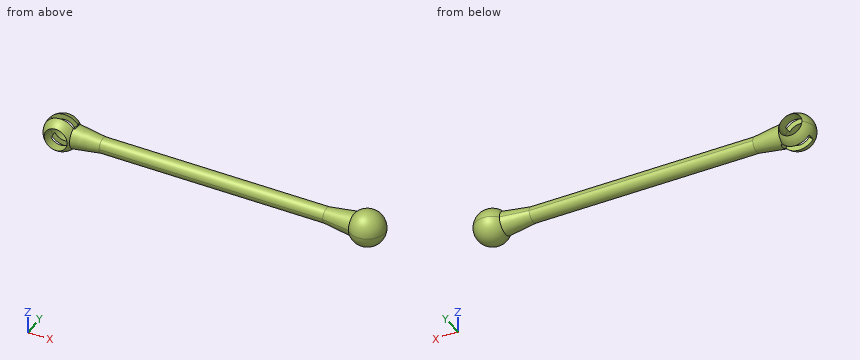
```python
from build123d import *
from build123d import SkipClean  # not in build123d's __all__

# Parameters (mm, degrees)
F2_W           = 30
F2_H           = 1.5
F3_ANGLE_BACK  = 90
F3_ANGLE       = 180
F5_ANGLE_BACK  = 90
F5_ANGLE       = 180
F7_ANGLE_BACK  = 90
F7_ANGLE       = 180
F9_R           = 2.25
F10_DEPTH      = 3.401
F10_DEPTH_BACK = 3.401
F12_DEPTH      = 0.75


with BuildPart() as f3:
    # F2 (on Front) → F3 (revolve)
    with BuildSketch(Plane.XZ, mode=Mode.PRIVATE) as f3_sk:
        with Locations((-15, 0.75)):
            Rectangle(F2_W, F2_H)
    revolve(f3_sk.sketch.rotate(Axis((0, 0, 0), (1, 0, 0)), -F3_ANGLE_BACK), axis=Axis((0, 0, 0), (1, 0, 0)), revolution_arc=F3_ANGLE)

    # F4 (on Front) → F5 (revolve)
    with BuildSketch(Plane.XZ, mode=Mode.PRIVATE) as f5_sk:
        with BuildLine():
            Line((-33.4, 0), (-26.6, 0))
            ThreePointArc((-26.6, 0), (-30, 3.4), (-33.4, 0))
        make_face()
    revolve(f5_sk.sketch.rotate(Axis((0, 0, 0), (1, 0, 0)), -F5_ANGLE_BACK), axis=Axis((0, 0, 0), (1, 0, 0)), revolution_arc=F5_ANGLE)

    # F6 (on Front) → F7 (revolve)
    with BuildSketch(Plane.XZ, mode=Mode.PRIVATE) as f7_sk:
        Polygon((-27.4509805807, 2.25), (-30, 2.25), (-30, 0), (-22, 0), (-22, 1.5), align=None)
    revolve(f7_sk.sketch.rotate(Axis((0, 0, 0), (1, 0, 0)), -F7_ANGLE_BACK), axis=Axis((0, 0, 0), (1, 0, 0)), revolution_arc=F7_ANGLE)

    # F8: F3 across plane


with BuildPart() as f3_1:
    add(f3.part, clean=False)
    add(f3.part.mirror(Plane.YZ), clean=False)

    # F9 (on Front) → F10 (cut, two sides)
    with BuildSketch(Plane.XZ) as f10_sk:
        with Locations((-30, 0)):
            Circle(F9_R)
    extrude(amount=-F10_DEPTH, mode=Mode.SUBTRACT)
    extrude(f10_sk.sketch, amount=F10_DEPTH_BACK, mode=Mode.SUBTRACT)

    # F11 (on Front) → F12 (cut, symmetric)
    with BuildSketch(Plane.XZ):
        Polygon((-34.15, 3.4), (-30.75, 0), (-29.25, 0), (-25.85, 3.4), align=None)
    extrude(amount=F12_DEPTH, both=True, mode=Mode.SUBTRACT)

    # F13: F3 across plane


with BuildPart() as f3_2:
    add(f3_1.part, clean=False)
    with SkipClean():  # cleaning this boolean's faces spoils the solid; the shape is the same uncleaned
        add(f3_1.part.mirror(Plane.XY), clean=False)


solid = f3_2.part
```
CAD build for the part. Positions are in the model's coordinates, mm. Round coordinates to 2 decimals unless told otherwise and drop trailing zeros. Write each loop counter-clockwise with the first axis right and the second up, starting at its lowest first coordinate (ties: lowest second). Pieces come first, ordered by that corner, then holes. Notation, with made-up numbers: (23.25, 7.25) -> (32.25, 7.25) arc R4 cw to (32.25, 13.25) -> close; hole circle Ø1 at (-6, 79.25). An arc over 180 degrees is marked (long way). Answer in a Markdown table with one row per item. Add a question column.
Item 1: Saw through at A-A, the plane x = -30. Write the cut outline in (y, z), then the cut area to 3 significant figures.
Item 2: Drop flat-ended pins along their axis: pin 1 Ø2 at (x, y) = (-7, -2) entering from +Z; pin 2 Ø2.5 at (x, z) = (-31, 2.5) entering from +Y; pin 3 Ø3 at (x, y) = (2, 2) entering from -Z. Give the stop position or say it passes through.
Item 3: Saw through at B-B, the plane x = 14. Write the cut outline in (y, z).
Item 4: Saw through at C-C, the plane x = 24. Write the cut outline in (y, z).
Item 5: Drill centre lines: line 1 (X direction, y = -2.25, z = -1.25); line 2 (X direction, y = -2, z = -1.5); line 3 (X direction, y = 0, z = 0.25). Where is each one in solid material? Low to high. Write a range as from..to.
Findings below:
| question | item | result |
|---|---|---|
| 1 | outline | (-2.55, -2.25) arc R3.4 ccw to (-0.75, -3.32) -> (-0.75, -2.25) -> close; (-2.55, 2.25) -> (-0.75, 2.25) -> (-0.75, 3.32) arc R3.4 ccw to start; (0.75, -3.32) arc R3.4 ccw to (2.55, -2.25) -> (0.75, -2.25) -> close; (0.75, 2.25) -> (2.55, 2.25) arc R3.4 ccw to (0.75, 3.32) -> close |
| 1 | area | 4.76 mm^2 |
| 2 | pin 1 | stops at z = 1.12 |
| 2 | pin 2 | stops at y = 2.55 |
| 2 | pin 3 | stops at z = -1.41 |
| 3 | outline | circle Ø3 at (0, 0) |
| 4 | outline | circle Ø3.55 at (0, 0) |
| 5 | line 1 | x = -32.22..-31.87, -28.13..-27.78, 27.78..32.22 |
| 5 | line 2 | x = -32.3..-31.68, -28.32..-27.7, 27.7..32.3 |
| 5 | line 3 | x = -33.39..-32.24, -27.76..33.39 |
